from build123d import *

# Parameters (mm, degrees)
BOSS_EXTRU_1_DEPTH       = 47
ESQUISSE3_R              = 2
ENL_V_MAT_EXTRU_2_DEPTH  = 50
ESQUISSE4_R              = 1.8
ESQUISSE4_R_2            = 7
ENL_V_MAT_EXTRU_3_DEPTH  = 5
BOSS_EXTRU_2_DEPTH       = 60
ESQUISSE11_W             = 8
ESQUISSE11_H             = 8
ESQUISSE11_R             = 2.3
ESQUISSE11_R_2           = 2.268048231
ESQUISSE11_W_2           = 6.384615385
ESQUISSE11_H_2           = 6.384615385
BOSS_EXTRU_6_DEPTH       = 6
ESQUISSE12_W             = 43
ESQUISSE12_H             = 12
ESQUISSE12_W_2           = 45
ENL_V_MAT_EXTRU_5_DEPTH  = 50
ESQUISSE13_W             = 5
ESQUISSE13_H             = 12
ENL_V_MAT_EXTRU_6_DEPTH  = 20
ESQUISSE25_R             = 13.4
ENL_V_MAT_EXTRU_8_DEPTH  = 2
ESQUISSE26_R             = 1.6
ENL_V_MAT_EXTRU_9_DEPTH  = 10
BOSS_EXTRU_7_DEPTH       = 2
ESQUISSE2_R              = 8
ENL_V_MAT_EXTRU_10_DEPTH = 60
ESQUISSE30_R             = 1.6
ENL_V_MAT_EXTRU_18_DEPTH = 10


with BuildPart() as part:
    # Esquisse1 → Boss.-Extru.1 (new body)
    with BuildSketch(Plane(origin=(0, 0, 0), x_dir=(1, 0, 0), z_dir=(0, 1, 0))):
        Polygon((-15, 0), (17, 0), (17, 50), (10, 50), (10, 6), (-10, 6), (-10, 106), (-15, 106), align=None)
    extrude(amount=BOSS_EXTRU_1_DEPTH)

    # Esquisse3 → Enlèv. mat.-Extru.2 (cut)
    with BuildSketch(Plane.ZY.offset(15)):
        with BuildLine():
            Line((-52, 30), (-52, 40))
            ThreePointArc((-52, 40), (-54, 38), (-56, 40))
            Line((-56, 40), (-56, 30))
            ThreePointArc((-56, 30), (-54, 32), (-52, 30))
        make_face()
        with Locations((-54, 40)):
            Circle(ESQUISSE3_R)
        with Locations((-54, 30)):
            Circle(ESQUISSE3_R)
    extrude(amount=-ENL_V_MAT_EXTRU_2_DEPTH, mode=Mode.SUBTRACT)

    # Esquisse4 → Enlèv. mat.-Extru.3 (cut)
    with BuildSketch(Plane(origin=(-10, 0, 0), x_dir=(0, 0, -1), z_dir=(1, 0, 0))):
        with Locations((85, 8)):
            Circle(ESQUISSE4_R)
        with Locations((95, 18)):
            Circle(ESQUISSE4_R)
        with Locations((75, 18)):
            Circle(ESQUISSE4_R)
        with Locations((85, 28)):
            Circle(ESQUISSE4_R)
        with Locations((85, 18)):
            Circle(ESQUISSE4_R_2)
    extrude(amount=-ENL_V_MAT_EXTRU_3_DEPTH, mode=Mode.SUBTRACT)

    # Esquisse4<4> → Boss.-Extru.2 (add)
    with BuildSketch(Plane(origin=(-10, 0, 0), x_dir=(0, 0, -1), z_dir=(1, 0, 0))):
        Polygon((94, 0), (106, 0), (106, 8.072261083), (94, 8.072261083), (94, 4.036130542), align=None)
        Polygon((67, 0), (76, 0), (76, 4), (76, 8.072261083), (67, 8.072261083), align=None)
        Polygon((76, 0), (94, 0), (94, 4.036130542), (76, 4), align=None)
    extrude(amount=-BOSS_EXTRU_2_DEPTH)

    # Esquisse11 → Boss.-Extru.6 (add)
    # profile 1 of 6: a face of its own
    with BuildSketch(Plane.XZ):
        with Locations((13, 4)):
            Rectangle(ESQUISSE11_W, ESQUISSE11_H)
        with Locations(Location((13, 4, 0), (0, 0, 270))):
            Circle(ESQUISSE11_R, mode=Mode.SUBTRACT)
    # profile 2 of 6: a face of its own
    with BuildSketch(Plane.XZ):
        Polygon((17, -58), (17, -50), (10, -50), (10, -46), (9, -46), (9, -58), align=None)
        with Locations(Location((13, -54, 0), (0, 0, 270))):
            Circle(ESQUISSE11_R, mode=Mode.SUBTRACT)
    # profile 3 of 6: a face of its own
    with BuildSketch(Plane.XZ):
        with Locations((-11, 4)):
            Rectangle(ESQUISSE11_W, ESQUISSE11_H)
        with Locations(Location((-11, 4, 0), (0, 0, 270))):
            Circle(ESQUISSE11_R_2, mode=Mode.SUBTRACT)
    # profile 4 of 6: a face of its own
    with BuildSketch(Plane.XZ):
        with Locations((-66, -63)):
            Rectangle(ESQUISSE11_W, ESQUISSE11_H)
        with Locations(Location((-66, -63, 0), (0, 0, 270))):
            Circle(ESQUISSE11_R, mode=Mode.SUBTRACT)
    # profile 5 of 6: a face of its own
    with BuildSketch(Plane.XZ):
        with Locations((-13.192307693, -109.192307693)):
            Rectangle(ESQUISSE11_W_2, ESQUISSE11_H_2)
        with Locations(Location((-13.192307692, -109.192307692, 0), (0, 0, 270))):
            Circle(ESQUISSE11_R, mode=Mode.SUBTRACT)
    # profile 6 of 6: a face of its own
    with BuildSketch(Plane.XZ):
        with Locations((-66.807692308, -109.192307693)):
            Rectangle(ESQUISSE11_W_2, ESQUISSE11_H_2)
        with Locations(Location((-66.807692308, -109.192307692, 0), (0, 0, 270))):
            Circle(ESQUISSE11_R, mode=Mode.SUBTRACT)
    extrude(amount=-BOSS_EXTRU_6_DEPTH)

    # Esquisse12 → Enlèv. mat.-Extru.5 (cut)
    with BuildSketch(Plane.ZY.offset(15)):
        with Locations((-84.5, 41)):
            Rectangle(ESQUISSE12_W, ESQUISSE12_H)
        with Locations((-22.5, 41)):
            Rectangle(ESQUISSE12_W_2, ESQUISSE12_H)
    extrude(amount=-ENL_V_MAT_EXTRU_5_DEPTH, mode=Mode.SUBTRACT)

    # Esquisse13 → Enlèv. mat.-Extru.6 (cut)
    with BuildSketch(Plane(origin=(17, 0, 0), x_dir=(0, 0, -1), z_dir=(1, 0, 0))):
        with Locations((47.5, 41)):
            Rectangle(ESQUISSE13_W, ESQUISSE13_H)
    extrude(amount=-ENL_V_MAT_EXTRU_6_DEPTH, mode=Mode.SUBTRACT)

    # Esquisse25 → Enlèv. mat.-Extru.8 (cut)
    with BuildSketch(Plane.ZY.offset(15)):
        with Locations((-85, 18)):
            Circle(ESQUISSE25_R)
    extrude(amount=-ENL_V_MAT_EXTRU_8_DEPTH, mode=Mode.SUBTRACT)

    # Esquisse26 → Enlèv. mat.-Extru.9 (cut)
    with BuildSketch(Plane(origin=(0, 35, 0), x_dir=(1, 0, 0), z_dir=(0, 1, 0))):
        with Locations(Location((13.5, 30, 0), (0, 0, 270))):
            Circle(ESQUISSE26_R)
    extrude(amount=-ENL_V_MAT_EXTRU_9_DEPTH, mode=Mode.SUBTRACT)

    # Esquisse27 → Boss.-Extru.7 (add)
    with BuildSketch(Plane.ZY.offset(15)):
        Polygon((0, 35), (0, 0), (-63, 0), (-63, 47), (-45, 47), (-45, 35), align=None)
    extrude(amount=BOSS_EXTRU_7_DEPTH)

    # Esquisse2 → Enlèv. mat.-Extru.10 (cut)
    with BuildSketch(Plane(origin=(17, 0, 0), x_dir=(0, 0, -1), z_dir=(1, 0, 0))):
        with Locations((30, 18)):
            Circle(ESQUISSE2_R)
    extrude(amount=-ENL_V_MAT_EXTRU_10_DEPTH, mode=Mode.SUBTRACT)

    # Esquisse30 → Enlèv. mat.-Extru.18 (cut)
    with BuildSketch(Plane(origin=(0, 35, 0), x_dir=(1, 0, 0), z_dir=(0, 1, 0))):
        with Locations(Location((-13.5, 30, 0), (0, 0, 270))):
            Circle(ESQUISSE30_R)
    extrude(amount=-ENL_V_MAT_EXTRU_18_DEPTH, mode=Mode.SUBTRACT)


solid = part.part
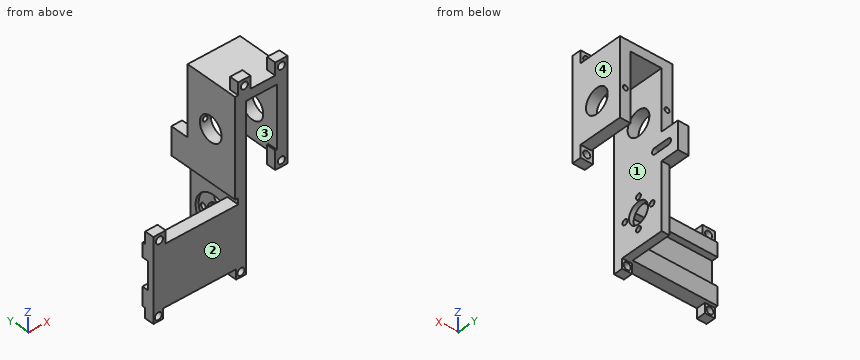
Verification items for the finished model (mm, model axes). Face numbers are marked on the shaded views. Coordinates: 2 decimals unless noted, no trailing zeros. Order: outer loops, then holes, each group sorted by start corner. A loop starts at its lowest first (then second) coordinate and runs counter-clockwise, first axis right, second up.
1. Release check for a two-part mould opening along X. For the marked faces 1, 2, 3 and 4 record: +X half, -X half, draft (parallel to the pull), parting line (faces both ways), or undercut.
Results found:
face 1: undercut
face 2: draft
face 3: undercut
face 4: +X half
2. Sectioned sample at C-C, the plane z = 4. Record the cut outline in (x, y), and give its area (3 significant figures).
Results found:
outline: (-15, 0) - (-13.27, 0) - (-13.27, 6) - (-15, 6) - close; (-8.73, 0) - (-7, 0) - (-7, 6) - (-8.73, 6) - close; (9, 0) - (10.7, 0) - (10.7, 6) - (9, 6) - close; (15.3, 0) - (17, 0) - (17, 6) - (15.3, 6) - close
area: 41.2 mm2
3. Sectioned sample at B-B, the plane y = 23. Record the cut outline in (x, z) (3 decimals).
Results found:
outline: (-17, -63) - (-15, -63) - (-15, -72.568) - (-13, -72.568) - (-13, -80.101) - (-10, -80.101) - (-10, -36.245) - (-17, -36.245) - close; (-17, -23.755) - (-10, -23.755) - (-10, -6) - (10, -6) - (10, -23.755) - (17, -23.755) - (17, 0) - (-17, 0) - close; (-15, -106) - (-10, -106) - (-10, -89.899) - (-13, -89.899) - (-13, -97.432) - (-15, -97.432) - close; (10, -50) - (17, -50) - (17, -36.245) - (10, -36.245) - close
4. Go/stop test with flat-tipped pins: pin 1 Ø3 at (y, z) = (3.5, -53) entering from -X; pin 2 Ø4 at (y, z) = (28, -85) entering from +X; pin 3 Ø5.5 at (x, z) = (13, -54) entering from -Y; pin 4 Ø2.5 at (x, y) = (-13, 32.5) entering from -Z. Record where each tip stops, or that it passes through.
Results found:
pin 1: stops at x = -17
pin 2: stops at x = -10
pin 3: stops at y = 0
pin 4: stops at z = -106
5. Sectioned sample at D-D, the plane z = -54. Record the cut outline in (x, y).
Results found:
outline: (-17, 0) - (-10, 0) - (-10, 28) - (-15, 28) - (-15, 42) - (-10, 42) - (-10, 47) - (-17, 47) - close; (9, 0) - (10.7, 0) - (10.7, 6) - (9, 6) - close; (15.3, 0) - (17, 0) - (17, 6) - (15.3, 6) - close
6. Scan lines: line 1 (X direction, y = 32.25, z = -30); line 2 (Y direction, x = -11.3, z = -85); line 3 (Z direction, x = 13.5, y = 29.25). Record each from-to range of solid material in increasing order.
Results found:
line 1: x = -17 to -15.1, -11.9 to -10, 10 to 11.9, 15.1 to 17
line 2: y = 0 to 6.2, 9.8 to 11, 25 to 26.2, 29.8 to 35
line 3: z = -50 to -31.6, -28.4 to 0
7. Sectioned sample at A-A, the plane z = -30. Record the cut outline in (x, y), and give its area (3 significant figures).
Results found:
outline: (-17, 0) - (-10, 0) - (-10, 10) - (-17, 10) - close; (-17, 26) - (-15.1, 26) - (-15.1, 35) - (-17, 35) - close; (-11.9, 26) - (-10, 26) - (-10, 35) - (-11.9, 35) - close; (10, 0) - (17, 0) - (17, 10) - (10, 10) - close; (10, 26) - (11.9, 26) - (11.9, 35) - (10, 35) - close; (15.1, 26) - (17, 26) - (17, 35) - (15.1, 35) - close
area: 208 mm2
